Source: CAD feature listing. Evaluate the final solid. Frame: model axes, mm. A direction names the side the tool comes from. Round coordinates to 2 decimals unless told otherwise and drop trailing zeros. Write each loop counter-clockwise with the first axis right and the second up, starting at its lowest first coordinate (ties: lowest second). Pieces come first, ordered by that corner, then holes.
from build123d import *

# Parameters (mm, degrees)
SKETCH_2_R               = 1.385
CUT_EXTRUDE_1_DEPTH      = 10
SKETCH_3_R               = 6.5
CUT_EXTRUDE_2_DEPTH      = 35
CUT_EXTRUDE_3_DEPTH      = 2
CUT_EXTRUDE_3_DEPTH_BACK = 10
SKETCH_5_R               = 1.425
SKETCH_11_W              = 11.431167052
SKETCH_11_H              = 3.4
EXTRUDE_3_DEPTH          = 35
SKETCH_13_R              = 1.425
CUT_EXTRUDE_4_DEPTH      = 16
SKETCH_14_R              = 0.877374271
CUT_EXTRUDE_5_DEPTH      = 12


with BuildPart() as part:
    # 草圖1 → 旋轉1 (revolve)
    with BuildSketch(Plane.XY, mode=Mode.PRIVATE) as revolve_1_sk:
        Polygon((0, 0), (0, 22), (4.87, 22), (10.87, 12.418858447), (14.37, 12.418858447), (20.37, 22), (25.24, 22), (25.24, 12.418858447), (35.24, 12.418858447), (35.24, 0), align=None)
    revolve(revolve_1_sk.sketch.rotate(Axis((-743.15639781, 0, 0), (1, 0, 0)), 90), axis=Axis((-743.15639781, 0, 0), (1, 0, 0)))

    # 草圖2 → 除料-伸長1 (cut)
    with BuildSketch(Plane(origin=(0, 12, 0), x_dir=(1, 0, 0), z_dir=(0, 1, 0))):
        with Locations(Location((30.456485429, 0, 0), (0, 0, 270))):
            Circle(SKETCH_2_R)
    extrude(amount=-CUT_EXTRUDE_1_DEPTH, mode=Mode.SUBTRACT)

    # 草圖3 → 除料-伸長2 (cut)
    with BuildSketch(Plane(origin=(35.24, 0, 0), x_dir=(0, 0, -1), z_dir=(1, 0, 0))):
        Circle(SKETCH_3_R)
    extrude(amount=-CUT_EXTRUDE_2_DEPTH, mode=Mode.SUBTRACT)

    # 草圖5 → 除料-伸長3 (cut, two sides: drawn at the far end of the back side and taken through both)
    with BuildSketch(Plane(origin=(0, 12, 0), x_dir=(1, 0, 0), z_dir=(0, 1, 0)).offset(-CUT_EXTRUDE_3_DEPTH_BACK)):
        with Locations(Location((30.456485429, 0, 0), (0, 0, 90))):
            Circle(SKETCH_5_R)
    extrude(amount=CUT_EXTRUDE_3_DEPTH + CUT_EXTRUDE_3_DEPTH_BACK, mode=Mode.SUBTRACT)

    # 草圖11 → 填料-伸長3 (add)
    with BuildSketch(Plane(origin=(35.24, 0, 0), x_dir=(0, 0, -1), z_dir=(1, 0, 0))):
        with Locations((-0.190572982, 5.582537257)):
            Rectangle(SKETCH_11_W, SKETCH_11_H)
    extrude(amount=-EXTRUDE_3_DEPTH)

    # 草圖13 → 除料-伸長4 (cut)
    with BuildSketch(Plane(origin=(0, 12, 0), x_dir=(1, 0, 0), z_dir=(0, 1, 0))):
        with Locations(Location((30.456485429, 0, 0), (0, 0, 90))):
            Circle(SKETCH_13_R)
    extrude(amount=-CUT_EXTRUDE_4_DEPTH, mode=Mode.SUBTRACT)

    # 草圖14 → 除料-伸長5 (cut)
    with BuildSketch(Plane.ZY):
        with Locations((-0.435299539, 17.00388826)):
            Circle(SKETCH_14_R)
    extrude(amount=-CUT_EXTRUDE_5_DEPTH, mode=Mode.SUBTRACT)


solid = part.part
1) Section query B-B on x = 11.5. Return the cut outline in (y, z), then the cut area to 3 significant figures.
Taken from the geometry:
outline: circle Ø24.84 at (0, 0); hole (3.88, -5.21) - (3.88, 5.21) arc R6.5 ccw (long way) to start
area: 371 mm2
2) Section query A-A on y = 0. Return the cut outline in (x, z), then the cut area to 3 significant figures.
Taken from the geometry:
outline: (0, -22) - (4.87, -22) - (10.87, -12.42) - (14.37, -12.42) - (20.37, -22) - (25.24, -22) - (25.24, -12.42) - (35.24, -12.42) - (35.24, -6.5) - (0.24, -6.5) - (0.24, 6.5) - (35.24, 6.5) - (35.24, 12.42) - (25.24, 12.42) - (25.24, 22) - (20.37, 22) - (14.37, 12.42) - (10.87, 12.42) - (4.87, 22) - (0, 22) - close
area: 722 mm2
3) Reachability of faces 1 (the face through (4.21, 16.15, -0.63)), 2 (the face through (12.645, -12.313, -1.617)), 3 (the face through (18, 3.883, 0)) from +Z, -Z, +X, -X, +Y, -Y: full face, straight path, thin tool, end or side. Return the list, or none.
Taken from the geometry:
face 1: -X
face 2: none
face 3: +X
4) Pull-direction query (Z, two-part tool) for faces 4 (the face through (29.044, 8.212, 0.186)), 5 (the face through (0.24, -1, 0)), 6 (the face through (0, 0, 0)), 7 (the face through (30.31, -12.313, -1.617)); classes: released by +Z, released by -Z, zero draft, split by the parting line, or undercut.
Taken from the geometry:
face 4: undercut
face 5: undercut
face 6: zero draft
face 7: split by the parting line
5) Contact query for flat-ended pins moving along their axis: P1, Ø6, axis at x = 24, z = 15, coming from the +Y side; P2, Ø1.5, axis at x = 30.5, y = -8, coming from the +Z side; P3, Ø5, axis at x = 21, z = -2.5, coming from the -Y side; P4, Ø1.5, axis at x = 12, y = 14.5, coming from the -Z side. Output: stop coordinate, or through.
Taken from the geometry:
P1: stops at y = 18.44
P2: stops at z = 10.08
P3: stops at y = -22
P4: passes through
6) Section query C-C on x = 6. Return the cut outline in (y, z).
Taken from the geometry:
outline: circle Ø40.39 at (0, 0); hole (3.88, -5.21) - (3.88, 5.21) arc R6.5 ccw (long way) to start; hole circle Ø1.75 at (17, -0.44)
7) Material intervals for line 1 (X direction, y = 6.25, z = 0); line 2 (X direction, y = -19, z = 1); line 3 (Y direction, x = 24, z = -6), sorted ascending.
Taken from the geometry:
line 1: x = 0 to 29.03, 31.88 to 35.24
line 2: x = 0 to 6.73, 18.51 to 25.24
line 3: y = -21.17 to -2.5, 2.5 to 21.17
